The model under review builds one solid part; all positions refer to its coordinate system, in mm. A direction names the side the tool comes from. Give positions to 0.01 mm unless a question says otherwise; leave off trailing zeros. Order: outer loops, then holes, each group sorted by start corner. A loop starts at its lowest first (then second) coordinate and runs counter-clockwise, first axis right, second up. Notation, with made-up numbers: (-8, 35) - (29, 35) arc R7 cw to (29, 46) - close; hole circle Ø1 at (24.5, 45). An arc over 180 degrees is marked (long way). Use CSV: the item, a comma, the result in double quotes. Start each with the question number.
1. For pin 1 (4.5 mm diameter, centred on x = -11.5, y = -3.5, fed in from +Z); pin 2 (1 mm diameter, centred on y = 17, z = 9, fed in from -X); pin 3 (5 mm diameter, centred on y = -1, z = 15, fed in from -X), all flat-tipped, find the tip position at first contact; note any pin that passes through.
2. To check wall thickness, follow line 1 (Z direction, x = 9, y = -13); line 2 (X direction, y = -21.5, z = 5.75); line 3 (X direction, y = -10.5, z = 17.25). State the ranges of each line that lie inside material, in increasing order. Write a range as [from, to].
3. Machinability: for faces 4 (the flat face through (0, 2.874, 10)), 5 (the cylindrical face through (20, 0, 2)), which of the approach directions +Z, -Z, +X, -X, +Y, -Y give a long, thin tool a straight path to every point of the face, cutting with its end or side? Answer none if there is none.
4. Draft analysis for pull direction X (two halves, no side actions). For faces 1 (the flat face through (13, 0, 5)), 2 (the cylindrical face through (-20, 0, 2)), 3 (the flat face through (2.977, 0, 10)), state which applies: released by +X, released by -X, zero draft, split by the parting line, or undercut.
5. Take a section at B-B, the plane x = 9. State the section outline as (y, z) points, then the cut area to 3 significant figures.
6. Take a section at A-A, the plane x = -16. State the section outline as (y, z) points.
```python
from build123d import *

# Parameters (mm, degrees)
F0_W     = 6
F0_H     = 6
F1_DEPTH = 20
F2_DEPTH = 5


with BuildPart() as f1:
    # F0 (on Top) → F1 (new body)
    with BuildSketch(Plane.XY):
        with BuildLine():
            add(Edge.make_bspline(
                [(0, 25), (-2.721114, 25), (-4.833477, 19.407151)],
                knots=[0, 0, 0, 0.682044, 0.682044, 0.682044], degree=2, weights=[1, 0.942413, 1]))
            add(Edge.make_bspline(
                [(-4.833477, 19.407151), (-12.163362, 0), (-4.833477, -19.407151)],
                knots=[0.682044, 0.682044, 0.682044, 2.459549, 2.459549, 2.459549], degree=2, weights=[1, 0.630381, 1]))
            add(Edge.make_bspline(
                [(-4.833477, -19.407151), (0, -32.204624), (4.833477, -19.407151)],
                knots=[2.459549, 2.459549, 2.459549, 3.823636, 3.823636, 3.823636], degree=2, weights=[1, 0.776286, 1]))
            add(Edge.make_bspline(
                [(4.833477, -19.407151), (12.163362, 0), (4.833477, 19.407151)],
                knots=[3.823636, 3.823636, 3.823636, 5.601142, 5.601142, 5.601142], degree=2, weights=[1, 0.630381, 1]))
            add(Edge.make_bspline(
                [(4.833477, 19.407151), (2.721114, 25), (0, 25)],
                knots=[5.601142, 5.601142, 5.601142, 6.283185, 6.283185, 6.283185], degree=2, weights=[1, 0.942413, 1]))
        make_face()
        with Locations((-0.022681, -0.126182)):
            Rectangle(F0_W, F0_H, mode=Mode.SUBTRACT)
    extrude(amount=F1_DEPTH)

    # F0 (on Top) → F2 (join)
    with BuildSketch(Plane.XY):
        with BuildLine():
            add(Edge.make_bspline(
                [(-4.833477, 19.407151), (-12.163362, 0), (-4.833477, -19.407151)],
                knots=[0.682044, 0.682044, 0.682044, 2.459549, 2.459549, 2.459549], degree=2, weights=[1, 0.630381, 1]))
            ThreePointArc((-4.833477, 19.407151), (-20, 0), (-4.833477, -19.407151))
        make_face()
        with BuildLine():
            add(Edge.make_bspline(
                [(0, 25), (-2.721114, 25), (-4.833477, 19.407151)],
                knots=[0, 0, 0, 0.682044, 0.682044, 0.682044], degree=2, weights=[1, 0.942413, 1]))
            add(Edge.make_bspline(
                [(-4.833477, 19.407151), (-12.163362, 0), (-4.833477, -19.407151)],
                knots=[0.682044, 0.682044, 0.682044, 2.459549, 2.459549, 2.459549], degree=2, weights=[1, 0.630381, 1]))
            add(Edge.make_bspline(
                [(-4.833477, -19.407151), (0, -32.204624), (4.833477, -19.407151)],
                knots=[2.459549, 2.459549, 2.459549, 3.823636, 3.823636, 3.823636], degree=2, weights=[1, 0.776286, 1]))
            add(Edge.make_bspline(
                [(4.833477, -19.407151), (12.163362, 0), (4.833477, 19.407151)],
                knots=[3.823636, 3.823636, 3.823636, 5.601142, 5.601142, 5.601142], degree=2, weights=[1, 0.630381, 1]))
            add(Edge.make_bspline(
                [(4.833477, 19.407151), (2.721114, 25), (0, 25)],
                knots=[5.601142, 5.601142, 5.601142, 6.283185, 6.283185, 6.283185], degree=2, weights=[1, 0.942413, 1]))
        make_face()
        with Locations((-0.022681, -0.126182)):
            Rectangle(F0_W, F0_H, mode=Mode.SUBTRACT)
        with BuildLine():
            add(Edge.make_bspline(
                [(4.833477, -19.407151), (12.163362, 0), (4.833477, 19.407151)],
                knots=[3.823636, 3.823636, 3.823636, 5.601142, 5.601142, 5.601142], degree=2, weights=[1, 0.630381, 1]))
            ThreePointArc((4.833477, -19.407151), (20, 0), (4.833477, 19.407151))
        make_face()
    extrude(amount=F2_DEPTH)


solid = f1.part
```
Determined:
1,pin 1,"stops at z = 5"
1,pin 2,"stops at x = -5.76"
1,pin 3,"stops at x = -7.67"
2,line 1,"z = [0, 5]"
2,line 2,"x = [-3.91, 3.91]"
2,line 3,"x = [-6.96, 6.96]"
3,face 4,"+Z, -Z"
3,face 5,"+Z, -Z, +X"
4,face 1,"zero draft"
4,face 2,"released by -X"
4,face 3,"undercut"
5,outline,"(-17.86, 0) - (17.86, 0) - (17.86, 5) - (-17.86, 5) - close"
5,area,"179 mm²"
6,outline,"(-12, 0) - (12, 0) - (12, 5) - (-12, 5) - close"
